```python
from build123d import *

# Parameters (mm, degrees)
F0_W      = 19.05
F0_H      = 38.1
F1_DEPTH  = 3.175
F2_R      = 1.651
F3_DEPTH  = 38.1
F4_W      = 10.7016550345
F4_H      = 25.4
F4_W_2    = 14.8274536716
F4_W_3    = 9.9113590219
F5_DEPTH  = 12.701
F6_R      = 5.08
F7_W      = 30.0603830089
F7_H      = 25.4
F8_DEPTH  = 9.525
F9_R      = 4.445
F9_R_2    = 1.651
F10_DEPTH = 3.175
F11_R     = 4.445
F11_R_2   = 1.651
F12_DEPTH = 3.175
F13_W     = 5.08
F13_H     = 25.4
F14_DEPTH = 3.175
F15_R     = 0.508


with BuildPart() as f1:
    # F0 (on Top) → F1 (new body)
    with BuildSketch(Plane.XY):
        Rectangle(F0_W, F0_H)
    extrude(amount=F1_DEPTH)

    # F2 (on face) → F3 (join, through all)
    with BuildSketch(Plane.XZ.offset(19.05)):
        with BuildLine():
            Line((25.5291087061, 0), (25.5291087061, 12.7))
            Line((25.5291087061, 12.7), (10.7016550345, 12.7))
            ThreePointArc((10.7016550345, 12.7), (10.1331167238, 12.6355533097), (9.5934291315, 12.4454836136))
            Line((9.5934291315, 12.4454836136), (-9.525, 3.175))
            Line((-9.525, 3.175), (9.525, 3.175))
            Line((9.525, 3.175), (9.525, 0))
            Line((9.525, 0), (14.3506696127, 0))
            Line((14.3506696127, 0), (25.5291087061, 0))
        make_face()
        with Locations((20.4010959715, 6.35)):
            Circle(F2_R, mode=Mode.SUBTRACT)
    extrude(amount=-F3_DEPTH)

    # F4 (on face) → F5 (cut, through all)
    with BuildSketch(Plane.XY.offset(12.7)):
        with Locations((5.3508275173, 0)):
            Rectangle(F4_W, F4_H)
        with Locations((18.1153818703, 0)):
            Rectangle(F4_W_2, F4_H)
        with Locations((30.4847882171, 0)):
            Rectangle(F4_W_3, F4_H)
    extrude(amount=-F5_DEPTH, mode=Mode.SUBTRACT)

    # F6
    f6_edges = [f1.edges().sort_by_distance(p)[0] for p in [
        (25.529109, -15.875, 12.7),
        (25.529109, -15.875, 0),
        (25.529109, 15.875, 0),
        (25.529109, 15.875, 12.7),
    ]]
    fillet(f6_edges, radius=F6_R)

    # F7 (on face) → F8 (cut, through all)
    with BuildSketch(Plane.XY.offset(12.7)):
        with Locations((-4.3285364699, 0)):
            Rectangle(F7_W, F7_H)
    extrude(amount=-F8_DEPTH, mode=Mode.SUBTRACT)

    # F9 (on face) → F10 (join)
    with BuildSketch(Plane(origin=(0, -12.7, 0), x_dir=(-1, 0, 0), z_dir=(0, 1, 0))):
        with Locations((-20.4010959715, 6.35)):
            Circle(F9_R)
        with Locations((-20.4588528723, 6.3269766979)):
            Circle(F9_R_2, mode=Mode.SUBTRACT)
    extrude(amount=F10_DEPTH)

    # F11 (on face) → F12 (join)
    with BuildSketch(Plane.XZ.offset(-12.7)):
        with Locations((20.4010959715, 6.35)):
            Circle(F11_R)
        with Locations((20.4010959715, 6.35)):
            Circle(F11_R_2, mode=Mode.SUBTRACT)
    extrude(amount=F12_DEPTH)

    # F13 (on face) → F14 (join, through all)
    with BuildSketch(Plane(origin=(0, 0, 0), x_dir=(1, 0, 0), z_dir=(0, 0, -1))):
        with Locations((2.54, 0)):
            Rectangle(F13_W, F13_H)
    extrude(amount=-F14_DEPTH)

    # F15
    f15_edges = [f1.edges().sort_by_distance(p)[0] for p in [
        (-2.2225, -12.7, 3.175),
        (-2.2225, 12.7, 3.175),
    ]]
    fillet(f15_edges, radius=F15_R)


solid = f1.part
```
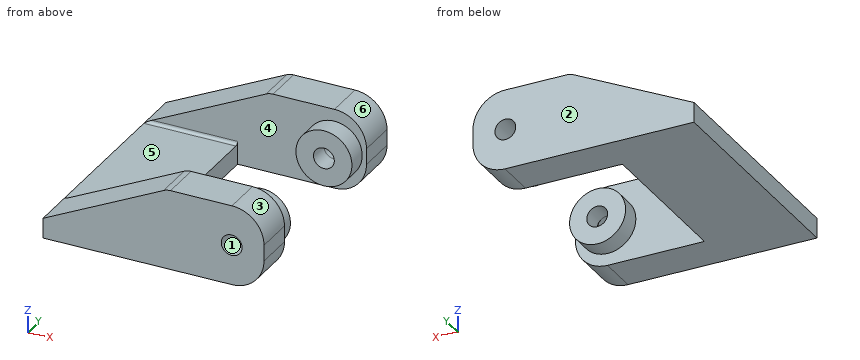
For this review, take the finished solid that the model builds, in its own axes (mm). Face numbers are marked on the shaded views. A direction names the side the tool comes from. Give positions to 0.01 mm unless a question says otherwise; leave off trailing zeros. Write each loop counter-clockwise with the first axis right and the second up, starting at its lowest first coordinate (ties: lowest second). Pieces come first, ordered by that corner, then holes. Notation, with made-up numbers: M -20,41 L 26,41 A22 ccw 26,75 Z; hole C 6,72 d1. An arc over 180 degrees is marked long. One line per item, written item: value.
1) For the marked faces 4, 5 and 6, list the 3-axis set-ups (+Z, -Z, +X, -X, +Y, -Y) from which the entire face can be reached by the end or side of a thin tool; tool diameter is ignored.
Results are:
face 4: none
face 5: +Z, -X
face 6: +Z, +X, +Y, -Y
2) For P1, Ø2.5, axis at x = 19, z = 6, coming from the +Y side; P2, Ø4, axis at y = -6, z = 1.5, coming from the +X side; P3, Ø7.5, axis at x = 0, y = 3.5, coming from the +Z side (3 decimals); P4, Ø3, axis at y = 13, z = 7, coming from the -X side, all flat-tipped, find the tip position at first contact; note any pin that passes through.
Results are:
P1: stops at y = 19.05
P2: stops at x = 5.08
P3: stops at z = 3.175
P4: stops at x = -4.73
3) The part is to be moulded in two halves that separate along X. For the marked faces 1, 2 and 3, say which applies: +X half, -X half, draft (parallel to the pull), parting line (faces both ways), or undercut.
Results are:
face 1: undercut
face 2: draft
face 3: +X half
4) For line 1 (Y direction, x = 22.5, z = 6) (3 decimals); line 2 (Y direction, x = 5, z = 4.75); line 3 (Z direction, x = 20, y = -10.5), list the stretches that pass through material, from the lowest coordinate up. Write a range as from..to.
Results are:
line 1: y = -19.05..-9.525, 9.525..19.05
line 2: y = -19.05..-12.7, 12.7..19.05
line 3: z = 1.92..4.74, 7.91..10.78
5) Take a section at A-A, the plane x = 16.5. Write out the cut boundary in (y, z) (3 decimals), then the cut area to 3 significant figures.
Results are:
outline: M -19.05,0 L -12.7,0 L -12.7,4.219 L -9.525,4.219 L -9.525,8.481 L -12.7,8.481 L -12.7,12.7 L -19.05,12.7 Z; M 9.525,4.219 L 12.7,4.219 L 12.7,0 L 19.05,0 L 19.05,12.7 L 12.7,12.7 L 12.7,8.481 L 9.525,8.481 Z
area: 188 mm²
6) Take a section at B-B, the plane y = 13.5. Write out the cut boundary in (x, z) (3 decimals).
Results are:
outline: M -9.525,0 L 20.449,0 A5.08 ccw 25.529,5.08 L 25.529,7.62 A5.08 ccw 20.449,12.7 L 10.702,12.7 A2.54 ccw 9.593,12.445 L -9.525,3.175 Z; hole C 20.401,6.35 d3.302
7) Take a section at C-C, the plane x = 2. Write out the cut boundary in (y, z) (3 decimals).
Results are:
outline: M -19.05,0 L 19.05,0 L 19.05,8.763 L 12.7,8.763 L 12.7,3.683 A0.508 cw 12.192,3.175 L -12.192,3.175 A0.508 cw -12.7,3.683 L -12.7,8.763 L -19.05,8.763 Z
8) Take a section at D-D, the plane y = 3.5. Write out the cut boundary in (x, z) (3 decimals), then the cut area to 3 significant figures.
Results are:
outline: M -9.525,0 L 5.08,0 L 5.08,3.175 L -9.525,3.175 Z
area: 46.4 mm²
